Read the model definition and answer for the solid it produces. Units are mm, in the model's axes. Face numbers are marked on the shaded views. A direction names the side the tool comes from. Coordinates: 2 decimals unless noted, no trailing zeros. Write each loop counter-clockwise with the first axis right and the second up, starting at its lowest first coordinate (ties: lowest second). Pieces come first, ordered by that corner, then holes.
(1) Given pin 1 (3.5 mm diameter, centred on x = 146.91, y = 10, fed in from +Z); pin 2 (0.6 mm diameter, centred on y = 3, z = 6.5, fed in from +X), each flat-ended and moving along its own axis, determine where each tip first touches the part or whether it passes through.
(2) Find the intervals of material crossed by probe 1 along X at (y, z) = (45, 5.5); probe 2 along Y at (x, z) = (142.5, 3.25); probe 3 along Y at (x, z) = (75, 8.5), in increasing order.
(3) Section D-D on x = 100.5 is taken. Write down the section's boundary in (y, z), then the cut area to 3 significant figures.
(4) Section A-A on x = 128.5 is taken. Write down the section's boundary in (y, z).
(5) The mould has two halves that part along X. Classify the marked faces 4, 5 and 6: +X half, -X half, draft (parallel to the pull), parting line (faces both ways), or undercut.
(6) Which of the six approach directions +Z, -Z, +X, -X, +Y, -Y give full straight-line access (tool end or side, diameter ignored) to the marked faces 1, 2 and 3?
(7) Section B-B on y = 22 is taken. Write down the section's boundary in (x, z).
(8) Section C-C on z = 8 is taken. State how many separate pieces and enclosed holes the cut face has, then the cut area to 3 significant figures.
from build123d import *

# Parameters (mm, degrees)
MODEL_R             = 2
MODEL_R_2           = 2.5
MODEL_R_3           = 2.55
MODEL_R_4           = 16.25
BOSS_EXTRUDE1_DEPTH = 10


with BuildPart() as part:
    # Model → Boss-Extrude1 (new body)
    with BuildSketch(Plane.XY):
        with BuildLine():
            Line((-13.089430894, 50), (-13.089430894, 6))
            ThreePointArc((-13.089430894, 6), (-9.401505079, 1.633399735), (-3.924279504, 0))
            Line((-3.924279504, 0), (34.910569106, 0))
            ThreePointArc((34.910569106, 0), (36.324782668, 0.585786438), (36.910569106, 2))
            Line((36.910569106, 2), (36.910569106, 4))
            ThreePointArc((36.910569106, 4), (37.496355543, 5.414213562), (38.910569106, 6))
            Line((38.910569106, 6), (103.910569106, 6))
            ThreePointArc((103.910569106, 6), (106.031889449, 5.121320344), (106.910569106, 3))
            ThreePointArc((106.910569106, 3), (107.789248762, 0.878679656), (109.910569106, 0))
            Line((109.910569106, 0), (146.910569106, 0))
            ThreePointArc((146.910569106, 0), (153.981636918, 2.928932188), (156.910569106, 10))
            Line((156.910569106, 10), (156.910569106, 50))
            ThreePointArc((156.910569106, 50), (153.981636918, 57.071067812), (146.910569106, 60))
            Line((146.910569106, 60), (116.910569106, 60))
            ThreePointArc((116.910569106, 60), (109.839501294, 57.071067812), (106.910569106, 50))
            Line((106.910569106, 50), (106.910569106, 40))
            ThreePointArc((106.910569106, 40), (103.981636918, 32.928932188), (96.910569106, 30))
            Line((96.910569106, 30), (46.910569106, 30))
            ThreePointArc((46.910569106, 30), (39.839501294, 32.928932188), (36.910569106, 40))
            Line((36.910569106, 40), (36.910569106, 50))
            ThreePointArc((36.910569106, 50), (33.981636918, 57.071067812), (26.910569106, 60))
            Line((26.910569106, 60), (-3.089430894, 60))
            ThreePointArc((-3.089430894, 60), (-10.160498706, 57.071067812), (-13.089430894, 50))
        make_face()
        with Locations((26.910569106, 50)):
            Circle(MODEL_R, mode=Mode.SUBTRACT)
        with Locations((26.910569106, 10)):
            Circle(MODEL_R, mode=Mode.SUBTRACT)
        with Locations((11.910569106, 30)):
            Circle(MODEL_R_2, mode=Mode.SUBTRACT)
        with Locations((146.910569106, 50)):
            Circle(MODEL_R, mode=Mode.SUBTRACT)
        with Locations((86.910569106, 18)):
            Circle(MODEL_R, mode=Mode.SUBTRACT)
        with Locations((146.910569106, 10)):
            Circle(MODEL_R, mode=Mode.SUBTRACT)
        with Locations((116.910569106, 10)):
            Circle(MODEL_R, mode=Mode.SUBTRACT)
        with Locations((46.910569106, 18)):
            Circle(MODEL_R, mode=Mode.SUBTRACT)
        with Locations((66.910569106, 18)):
            Circle(MODEL_R, mode=Mode.SUBTRACT)
        with Locations((116.910569106, 50)):
            Circle(MODEL_R, mode=Mode.SUBTRACT)
        with Locations((11.910569106, 18)):
            Circle(MODEL_R_3, mode=Mode.SUBTRACT)
        with Locations((-3.089430894, 10)):
            Circle(MODEL_R, mode=Mode.SUBTRACT)
        with Locations((-3.089430894, 50)):
            Circle(MODEL_R, mode=Mode.SUBTRACT)
        with Locations((131.910569106, 30)):
            Circle(MODEL_R_4, mode=Mode.SUBTRACT)
    extrude(amount=BOSS_EXTRUDE1_DEPTH)


solid = part.part
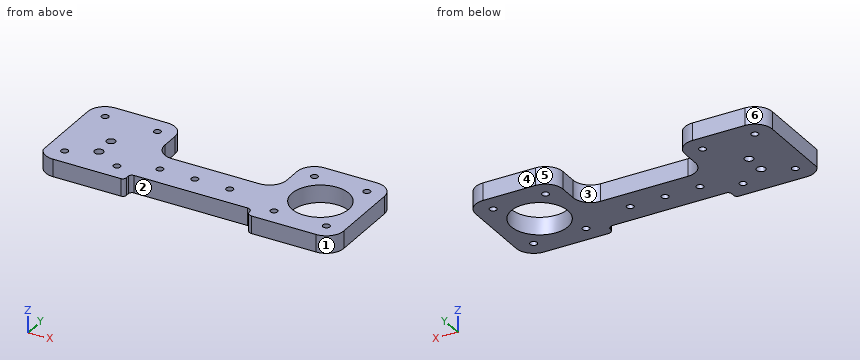
Response:
1. pin 1: passes through
1. pin 2: stops at x = 154.33
2. probe 1: x = -13.09 to 36.91, 106.91 to 125.66, 138.16 to 156.91
2. probe 2: y = 0 to 17.67, 42.33 to 60
2. probe 3: y = 6 to 30
3. outline: (6, 0) - (30.67, 0) - (30.67, 10) - (6, 10) - close
3. area: 247 mm2
4. outline: (0, 0) - (14.11, 0) - (14.11, 10) - (0, 10) - close; (45.89, 0) - (60, 0) - (60, 10) - (45.89, 10) - close
5. face 4: draft
5. face 5: undercut
5. face 6: -X half
6. face 1: +Z, -Z, +X, -Y
6. face 2: +Z, -Z, -Y
6. face 3: +Z, -Z, +Y
7. outline: (-13.09, 0) - (117.77, 0) - (117.77, 10) - (-13.09, 10) - close; (146.05, 0) - (156.91, 0) - (156.91, 10) - (146.05, 10) - close
8. separate pieces: 1
8. enclosed holes: 14
8. area: 6,590 mm2
